from build123d import *

# Parameters (mm, degrees)
SKETCH072_R           = 12.25
PAD027_DEPTH          = 10
FILLET040_R           = 0.5
PAD030_DEPTH          = 7.5
SKETCH063_R           = 32.89
SKETCH063_R_2         = 18.75
POCKET020_DEPTH       = 94.210561
POLARPATTERN006_COUNT = 8


with BuildPart() as part:
    # Sketch072 → Pad027 (new body)
    with BuildSketch(Plane.XY):
        Circle(SKETCH072_R)
    extrude(amount=PAD027_DEPTH)

    # Fillet040
    fillet040_edges = [part.edges().sort_by_distance(p)[0] for p in [
        (-12.25, 0, 10),
        (-12.25, 0, 0),
    ]]
    fillet(fillet040_edges, radius=FILLET040_R)

    # Sketch085 (on DatumPlane) → Pad030 (join, symmetric)
    with BuildSketch(Plane(origin=(0, 13, -2), x_dir=(1, 0, 0), z_dir=(0, -1, 0))):
        with BuildLine():
            ThreePointArc((5.3, 10), (-1.072659, 8.299055), (-5, 3))
            ThreePointArc((5.3, 10), (-0.742753, 7.813623), (-5, 3))
        make_face()
    pad030 = extrude(amount=PAD030_DEPTH, both=True)

    # Sketch063 (on Face7 of Pad030) → Pocket020 (cut, through all)
    with BuildSketch(Plane.XY.offset(10)):
        Circle(SKETCH063_R)
        Circle(SKETCH063_R_2, mode=Mode.SUBTRACT)
    pocket020 = extrude(amount=-POCKET020_DEPTH, mode=Mode.SUBTRACT)

    # PolarPattern006: Pad030, Pocket020 ×8 about axis
    polarpattern006_axis = Axis((0, 0, 0), (0, 0, 1))
    for i in range(1, POLARPATTERN006_COUNT):
        add(pad030.rotate(polarpattern006_axis, i * 360 / POLARPATTERN006_COUNT))
        add(pocket020.rotate(polarpattern006_axis, i * 360 / POLARPATTERN006_COUNT), mode=Mode.SUBTRACT)


solid = part.part
Part model, mm, in its own coordinate system. A direction names the side the tool comes from. Coordinates: 2 decimals unless noted, no trailing zeros. Loops run counter-clockwise (first coordinate to the right, second up) from the corner with the lowest first, then second, coordinate; pieces in that order, holes last. Notation, with made-up numbers: (30.25, 66) -> (65.25, 66) arc R9 cw to (65.25, 79) -> close; hole circle Ø4 at (-17, 78). An arc over 180 degrees is marked (long way). Use a Markdown table: item, result. Add a question column.
Item 1: Band-saw the part on B-B on y = 0. Write the cut outline in (x, z).
Item 2: Which spindle directions (+Z, -Z, +X, -X, +Y, -Y) get a long thin tool onto all of the face, cutting with end or side? Do faces 5 (the cylindrical face through (12.55, 13.93, 5.84)), 6 (the cylindrical face through (-9.03, 8.28, 4.94)). Say none if no direction does.
Item 3: Flat gauge pins, fed straight in: P1, Ø2, axis at x = -7.5, z = 8.5, coming from the -Y side; P2, Ø4, axis at x = 13.5, z = 6.5, coming from the +Y side; P3, Ø1, axis at x = -5.5, z = 5.5, coming from the -Y side. Where does each tip first touch, or does it go through?
Item 4: Probe probe 1 along Y at (x, z) = (-12.5, 2); probe 2 along Y at (x, z) = (14.5, 4.75); probe 3 along X at (y, z) = (8.5, 5). List the from-to ranges inside material, lowest first.
Item 5: Pull direction Y, two halves, no side cores. Call faces 1 (the cylindrical face through (-10.97, 10.02, 5.86)), 2 (the cylindrical face through (13.7, -12.8, 6.1)), 3 (the cylindrical face through (-10.02, -10.97, 5.86)), 4 (the flat face through (0, 0, 0)): +Y half, -Y half, draft (parallel to the pull), parting line (faces both ways), or undercut.
Item 6: Band-saw the part on D-D on z = 8.75. Write the cut outline in (x, y).
Geometry says:
| question | item | result |
|---|---|---|
| 1 | outline | (-18.75, 6.28) -> (-12.25, 6.28) -> (-12.25, 0.5) arc R0.5 ccw to (-11.75, 0) -> (11.75, 0) arc R0.5 ccw to (12.25, 0.5) -> (12.25, 6.28) -> (18.75, 6.28) -> (18.75, 6.93) -> (12.25, 6.93) -> (12.25, 9.5) arc R0.5 ccw to (11.75, 10) -> (-11.75, 10) arc R0.5 ccw to (-12.25, 9.5) -> (-12.25, 6.93) -> (-18.75, 6.93) -> close |
| 2 | face 5 | +Z, -Z, +X, +Y |
| 2 | face 6 | none |
| 3 | P1 | y = -10.38 |
| 3 | P2 | y = 14.62 |
| 3 | P3 | y = -11.18 |
| 4 | probe 1 | -4.63 to -4.43, 5.95 to 6.24 |
| 4 | probe 2 | -11.52 to -10.46, 2.1 to 2.86 |
| 4 | probe 3 | -12.21 to -11.07, -8.82 to 8.82 |
| 5 | face 1 | +Y half |
| 5 | face 2 | -Y half |
| 5 | face 3 | undercut |
| 5 | face 4 | draft |
| 6 | outline | circle Ø24.5 at (0, 0) |
